Work out the finished part from the listing and answer in its coordinate system (mm). A direction names the side the tool comes from. Coordinates: 2 decimals unless noted, no trailing zeros. Write each loop counter-clockwise with the first axis right and the second up, starting at its lowest first coordinate (ties: lowest second). Pieces come first, ordered by that corner, then holes. Notation, with made-up numbers: (-18, 29.25) - (-3, 29.25) arc R33 cw to (-3, 62.25) - close; hole circle Ø6 at (-33, 38.25). An arc over 180 degrees is marked (long way). Use one line per item in the form item = value. Start each with the question number.
Item 1: Consider probe 1 along X at (y, z) = (-0.9, 162.97); probe 2 along Y at (x, z) = (83.5, 147.5); probe 3 along Y at (x, z) = (92, 138). Determine where each line is inside the solid, lowest interval first.
Item 2: For faces 4 (the flat face through (67, 35, 137.014)), 5 (the flat face through (67, 34, 138.614)), determine the directions among +Z, -Z, +X, -X, +Y, -Y from which every point of the face is accessible in a straight line to the end or side of a thin tool.
Item 3: A cutting plane is placed at C-C (x = 97.28). Write down the section's boundary in (y, z), then the cut area to 3 significant figures.
Item 4: A cutting plane is placed at D-D (y = 21). Write down the section's boundary in (x, z).
Item 5: Determine the mould class of faces 1 (the cylindrical face through (94.681, 63.115, 137.803)), 2 (the flat face through (67, -1.6, 158)), 3 (the cylindrical face through (37.78, 88.67, 164.41)) for opening direction Y: released by +Y, released by -Y, zero draft, split by the parting line, or undercut.
Item 6: A cutting plane is placed at B-B (z = 151). Write down the section's boundary in (x, y).
Item 7: Given pin 1 (1.3 mm diameter, centred on x = 68.5, z = 137.5, fed in from +Y); pin 2 (10 mm diameter, centred on y = 20.5, z = 146.5, fed in from +X); pin 3 (5.5 mm diameter, centred on x = 42.69, y = 43.94, fed in from -Z); pin 4 (1 mm diameter, centred on x = 99.5, y = 24.5, fed in from +Z), each flat-ended and moving along its own axis, determine where each tip first touches the part or whether it passes through.
Item 8: A cutting plane is placed at A-A (x = 74.5). Write down the section's boundary in (y, z), then the cut area to 3 significant figures.
from build123d import *

# Parameters (mm, degrees)
SKETCH1_W                    = 135.38
SKETCH1_H                    = 188.37
SKETCH1_R                    = 1.4732
SKETCH1_R_2                  = 2.155
SKETCH1_W_2                  = 30
SKETCH1_H_2                  = 20
BASE_FLANGE1_DEPTH           = 1.6002
SKETCHED_BEND1_OUTLINE_W     = 135.38
SKETCHED_BEND1_OUTLINE_H     = 1.6002
SKETCHED_BEND1_DEPTH         = 137.314310973
SKETCHED_START               = 164.4432001
SKETCHED_BEND1_2_OUTLINE_W   = 135.38
SKETCHED_BEND1_2_OUTLINE_H   = 1.6002
SKETCHED_BEND1_2_DEPTH       = 23.9267999
SKETCHED_START_2             = 139.935207433
SKETCHED_BEND1_3_OUTLINE_W   = 135.38
SKETCHED_BEND1_3_OUTLINE_H   = 1.6002
SKETCHED_BEND1_3_DEPTH       = 21.561592467
SKETCHED_START_3             = 138.466703893
SKETCHED_BEND1_4_OUTLINE_W   = 135.38
SKETCHED_BEND1_4_OUTLINE_H   = 87.881185133
SKETCHED_BEND1_4_OUTLINE_R   = 2.155
SKETCHED_BEND1_4_OUTLINE_W_2 = 30
SKETCHED_BEND1_4_OUTLINE_H_2 = 20
SKETCHED_BEND1_4_DEPTH       = 0.14770354
SKETCHED_START_4             = 137.014207433
SKETCHED_BEND1_5_OUTLINE_W   = 135.38
SKETCHED_BEND1_5_OUTLINE_H   = 87.881185133
SKETCHED_BEND1_5_OUTLINE_R   = 2.155
SKETCHED_BEND1_5_OUTLINE_W_2 = 30
SKETCHED_BEND1_5_OUTLINE_H_2 = 20
SKETCHED_BEND1_5_DEPTH       = 2.921
SKETCHED_START_5             = 137.314310973
SKETCHED_BEND1_6_OUTLINE_W   = 135.38
SKETCHED_BEND1_6_OUTLINE_H   = 1.6002
SKETCHED_BEND1_6_DEPTH       = 27.128889127
SKETCHED_BEND1_7_DEPTH       = 135.38
SKETCHED_START_6             = 87
SKETCHED_BEND1_8_OUTLINE_R   = 1.4732
SKETCHED_BEND1_8_DEPTH       = 2.481385133


with BuildPart() as part:
    # Base-Flange1: sheet metal written as solids
    # Sketch1 → Base-Flange1 (new body)
    with BuildSketch(Plane(origin=(0, 0, 0), x_dir=(1, 0, 0), z_dir=(0, 1, 0))):
        with Locations((67.69, -94.185)):
            Rectangle(SKETCH1_W, SKETCH1_H)
        with Locations(Location((38.1, -25.4, 0), (0, 0, 270))):
            Circle(SKETCH1_R, mode=Mode.SUBTRACT)
        with Locations(Location((97.28, -25.4, 0), (0, 0, 270))):
            Circle(SKETCH1_R, mode=Mode.SUBTRACT)
        with Locations(Location((97.28, -162.97, 0), (0, 0, 90))):
            Circle(SKETCH1_R, mode=Mode.SUBTRACT)
        with Locations(Location((38.1, -162.97, 0), (0, 0, 90))):
            Circle(SKETCH1_R, mode=Mode.SUBTRACT)
        with Locations(Location((67.69, -25.4, 0), (0, 0, 270))):
            Circle(SKETCH1_R, mode=Mode.SUBTRACT)
        with Locations(Location((67.69, -162.97, 0), (0, 0, 270))):
            Circle(SKETCH1_R, mode=Mode.SUBTRACT)
        with Locations(Location((42.69, -94.185, 0), (0, 0, 270))):
            Circle(SKETCH1_R_2, mode=Mode.SUBTRACT)
        with Locations(Location((92.69, -94.185, 0), (0, 0, 270))):
            Circle(SKETCH1_R_2, mode=Mode.SUBTRACT)
        with Locations(Location((42.69, -74.185, 0), (0, 0, 270))):
            Circle(SKETCH1_R_2, mode=Mode.SUBTRACT)
        with Locations(Location((92.69, -74.185, 0), (0, 0, 270))):
            Circle(SKETCH1_R_2, mode=Mode.SUBTRACT)
        with Locations((67.69, -92.185)):
            Rectangle(SKETCH1_W_2, SKETCH1_H_2, mode=Mode.SUBTRACT)
    extrude(amount=-BASE_FLANGE1_DEPTH)

    # Sketched Bend1: read off the stored shape, not the designer's step
    # Sketched Bend1 outline → Sketched Bend1 (cut)
    with BuildSketch(Plane.XY):
        with Locations((67.69, -0.8001)):
            Rectangle(SKETCHED_BEND1_OUTLINE_W, SKETCHED_BEND1_OUTLINE_H)
    extrude(amount=SKETCHED_BEND1_DEPTH, mode=Mode.SUBTRACT)

    # Sketched Bend1 4 outline → Sketched Bend1 4 (add)
    with BuildSketch(Plane.XY.offset(SKETCHED_START_3)):
        with Locations((67.69, 43.940592567)):
            Rectangle(SKETCHED_BEND1_4_OUTLINE_W, SKETCHED_BEND1_4_OUTLINE_H)
        with Locations((42.69, 43.940592567)):
            Circle(SKETCHED_BEND1_4_OUTLINE_R, mode=Mode.SUBTRACT)
        with Locations((42.69, 63.940592567)):
            Circle(SKETCHED_BEND1_4_OUTLINE_R, mode=Mode.SUBTRACT)
        with Locations((67.69, 45.940592567)):
            Rectangle(SKETCHED_BEND1_4_OUTLINE_W_2, SKETCHED_BEND1_4_OUTLINE_H_2, mode=Mode.SUBTRACT)
        with Locations((92.69, 43.940592567)):
            Circle(SKETCHED_BEND1_4_OUTLINE_R, mode=Mode.SUBTRACT)
        with Locations((92.69, 63.940592567)):
            Circle(SKETCHED_BEND1_4_OUTLINE_R, mode=Mode.SUBTRACT)
    extrude(amount=SKETCHED_BEND1_4_DEPTH)



with BuildPart() as body_2:
    # Sketched Bend1 2 outline → Sketched Bend1 2 (new body)
    with BuildSketch(Plane.XY.offset(SKETCHED_START)):
        with Locations((67.69, 88.681285133)):
            Rectangle(SKETCHED_BEND1_2_OUTLINE_W, SKETCHED_BEND1_2_OUTLINE_H)
    extrude(amount=SKETCHED_BEND1_2_DEPTH)


with BuildPart() as body_3:
    # Sketched Bend1 3 outline → Sketched Bend1 3 (new body)
    with BuildSketch(Plane.XY.offset(SKETCHED_START_2)):
        with Locations((67.69, 88.681285133)):
            Rectangle(SKETCHED_BEND1_3_OUTLINE_W, SKETCHED_BEND1_3_OUTLINE_H)
    extrude(amount=SKETCHED_BEND1_3_DEPTH)


with BuildPart() as part_1:
    add(part.part)

    add(body_3.part)  # Sketched Bend1 5 merges body 3
    # Sketched Bend1 5 outline → Sketched Bend1 5 (add)
    with BuildSketch(Plane.XY.offset(SKETCHED_START_4)):
        with Locations((67.69, 43.940592567)):
            Rectangle(SKETCHED_BEND1_5_OUTLINE_W, SKETCHED_BEND1_5_OUTLINE_H)
        with Locations((42.69, 43.940592567)):
            Circle(SKETCHED_BEND1_5_OUTLINE_R, mode=Mode.SUBTRACT)
        with Locations((92.69, 43.940592567)):
            Circle(SKETCHED_BEND1_5_OUTLINE_R, mode=Mode.SUBTRACT)
        with Locations((42.69, 63.940592567)):
            Circle(SKETCHED_BEND1_5_OUTLINE_R, mode=Mode.SUBTRACT)
        with Locations((67.69, 45.940592567)):
            Rectangle(SKETCHED_BEND1_5_OUTLINE_W_2, SKETCHED_BEND1_5_OUTLINE_H_2, mode=Mode.SUBTRACT)
        with Locations((92.69, 63.940592567)):
            Circle(SKETCHED_BEND1_5_OUTLINE_R, mode=Mode.SUBTRACT)
    extrude(amount=SKETCHED_BEND1_5_DEPTH)


    add(body_2.part)  # Sketched Bend1 6 merges body 2
    # Sketched Bend1 6 outline → Sketched Bend1 6 (add)
    with BuildSketch(Plane.XY.offset(SKETCHED_START_5)):
        with Locations((67.69, 88.681285133)):
            Rectangle(SKETCHED_BEND1_6_OUTLINE_W, SKETCHED_BEND1_6_OUTLINE_H)
    extrude(amount=SKETCHED_BEND1_6_DEPTH)

    # Sketched Bend1 7 outline → Sketched Bend1 7 (cut)
    with BuildSketch(Plane.YZ):
        with BuildLine():
            ThreePointArc((89.481385133, 139.935207433), (88.62584404, 137.869748526), (86.560385133, 137.014207433))
            Line((86.560385133, 137.014207433), (87.881185133, 137.014207433))
            Line((87.881185133, 137.014207433), (87.881185133, 137.314310973))
            Line((87.881185133, 137.314310973), (89.481385133, 137.314310973))
            Line((89.481385133, 137.314310973), (89.481385133, 139.935207433))
        make_face()
        with BuildLine():
            Line((0, 137.014207433), (1.3208, 137.014207433))
            ThreePointArc((1.3208, 137.014207433), (-0.744658907, 137.869748526), (-1.6002, 139.935207433))
            Line((-1.6002, 139.935207433), (-1.6002, 137.314310973))
            Line((-1.6002, 137.314310973), (0, 137.314310973))
            Line((0, 137.314310973), (0, 137.014207433))
        make_face()
        with BuildLine():
            ThreePointArc((86.560385133, 138.614407433), (87.49433177, 139.001260796), (87.881185133, 139.935207433))
            Line((87.881185133, 139.935207433), (0, 139.935207433))
            ThreePointArc((0, 139.935207433), (0.386853363, 139.001260796), (1.3208, 138.614407433))
            Line((1.3208, 138.614407433), (86.560385133, 138.614407433))
        make_face()
    extrude(amount=SKETCHED_BEND1_7_DEPTH, mode=Mode.SUBTRACT)

    # Sketched Bend1 8 outline → Sketched Bend1 8 (cut)
    with BuildSketch(Plane(origin=(0, 0, 0), x_dir=(1, 0, 0), z_dir=(0, 1, 0)).offset(SKETCHED_START_6)):
        with Locations((67.69, -162.97)):
            Circle(SKETCHED_BEND1_8_OUTLINE_R)
        with Locations((97.28, -162.97)):
            Circle(SKETCHED_BEND1_8_OUTLINE_R)
        with Locations((38.1, -162.97)):
            Circle(SKETCHED_BEND1_8_OUTLINE_R)
    extrude(amount=SKETCHED_BEND1_8_DEPTH, mode=Mode.SUBTRACT)


solid = part_1.part
Answer:
q1.probe_1 = 0 to 36.63, 39.57 to 66.22, 69.16 to 95.81, 98.75 to 135.38
q1.probe_2 = -1.6 to 0, 87.88 to 89.48
q1.probe_3 = -0.87 to 41.9, 45.98 to 61.9, 65.98 to 88.75
q2.face_4 = -Z, +X, -X, +Y, -Y
q2.face_5 = +Z, +X, -X
q3.outline = (-1.6, 139.94) arc R2.92 ccw to (1.32, 137.01) - (86.56, 137.01) arc R2.92 ccw to (89.48, 139.94) - (89.48, 161.5) - (87.88, 161.5) - (87.88, 139.94) arc R1.32 cw to (86.56, 138.61) - (1.32, 138.61) arc R1.32 cw to (0, 139.94) - (0, 161.5) - (-1.6, 161.5) - close; (-1.6, 164.44) - (0, 164.44) - (0, 188.37) - (-1.6, 188.37) - close; (87.88, 164.44) - (89.48, 164.44) - (89.48, 188.37) - (87.88, 188.37) - close
q3.area = 293 mm²
q4.outline = (0, 137.01) - (135.38, 137.01) - (135.38, 138.61) - (0, 138.61) - close
q5.face_1 = undercut
q5.face_2 = released by -Y
q5.face_3 = zero draft
q6.outline = (0, -1.6) - (135.38, -1.6) - (135.38, 0) - (0, 0) - close; (0, 87.88) - (135.38, 87.88) - (135.38, 89.48) - (0, 89.48) - close
q7.pin_1 = 88.87
q7.pin_2 = through
q7.pin_3 = 137.01
q7.pin_4 = 138.61
q8.outline = (-1.6, 139.94) arc R2.92 ccw to (1.32, 137.01) - (35.94, 137.01) - (35.94, 138.61) - (1.32, 138.61) arc R1.32 cw to (0, 139.94) - (0, 188.37) - (-1.6, 188.37) - close; (55.94, 137.01) - (86.56, 137.01) arc R2.92 ccw to (89.48, 139.94) - (89.48, 188.37) - (87.88, 188.37) - (87.88, 139.94) arc R1.32 cw to (86.56, 138.61) - (55.94, 138.61) - close
q8.area = 270 mm²
